from build123d import *

# Parameters (mm, degrees)
SKETCH_W          = 20
SKETCH_H          = 9
PAD_DEPTH         = 0.5
PAD001_DEPTH      = 3
PAD001_FACE6_W    = 9
PAD001_FACE6_H    = 0.5
PAD002_DEPTH      = 160
PAD003_DEPTH      = 3
SKETCH003_R       = 1.7
POCKET_DEPTH      = 5
SKETCH004_W       = 9
SKETCH004_H       = 3.5
POCKET001_DEPTH   = 10
SKETCH005_W       = 9
SKETCH005_H       = 3.5
POCKET002_DEPTH   = 5
POCKET002_FACE2_W = 9
POCKET002_FACE2_H = 165
POCKET002_FACE2_R = 1.7
POCKET003_DEPTH   = 0.1
POCKET004_DEPTH   = 0.1
SKETCH006_R       = 1.9
POCKET005_DEPTH   = 5
POCKET005_FACE6_W = 164.9
POCKET005_FACE6_H = 0.4
POCKET006_DEPTH   = 0.1
POCKET006_FACE1_W = 164.9
POCKET006_FACE1_H = 0.4
POCKET007_DEPTH   = 0.1
POCKET008_DEPTH   = 5


with BuildPart() as part:
    # Sketch → Pad (new body)
    with BuildSketch(Plane.XY):
        Rectangle(SKETCH_W, SKETCH_H)
    extrude(amount=PAD_DEPTH)

    # Sketch001 (on Face6 of Pad) → Pad001 (join)
    with BuildSketch(Plane.XY.offset(0.5)):
        with BuildLine():
            ThreePointArc((-3.6, 2.4), (-6, 0), (-3.6, -2.4))
            Line((-3.6, -2.4), (3.6, -2.4))
            ThreePointArc((3.6, -2.4), (6, 0), (3.6, 2.4))
            Line((-3.6, 2.4), (3.6, 2.4))
        make_face()
    extrude(amount=PAD001_DEPTH)

    # Pad001 Face6 → Pad002 (add)
    with BuildSketch(Plane(origin=(10, 0, 0.25), x_dir=(0, -1, 0), z_dir=(1, 0, 0))):
        Rectangle(PAD001_FACE6_W, PAD001_FACE6_H)
    extrude(amount=PAD002_DEPTH)

    # Sketch002 (on Face6 of Pad002) → Pad003 (join)
    with BuildSketch(Plane.XY.offset(0.5)):
        with BuildLine():
            ThreePointArc((16.6, 2.4), (14.2, 0), (16.6, -2.4))
            Line((16.6, -2.4), (43.8, -2.4))
            ThreePointArc((43.8, -2.4), (46.2, 0), (43.8, 2.4))
            Line((16.6, 2.4), (43.8, 2.4))
        make_face()
        with BuildLine():
            ThreePointArc((56.74, 2.4), (54.34, 0), (56.74, -2.4))
            Line((56.74, -2.4), (83.94, -2.4))
            ThreePointArc((83.94, -2.4), (86.34, 0), (83.94, 2.4))
            Line((56.74, 2.4), (83.94, 2.4))
        make_face()
        with BuildLine():
            ThreePointArc((96.88, 2.4), (94.48, 0), (96.88, -2.4))
            Line((96.88, -2.4), (124.08, -2.4))
            ThreePointArc((124.08, -2.4), (126.48, 0), (124.08, 2.4))
            Line((96.88, 2.4), (124.08, 2.4))
        make_face()
        with BuildLine():
            ThreePointArc((137.02, 2.4), (134.62, 0), (137.02, -2.4))
            Line((137.02, -2.4), (164.22, -2.4))
            ThreePointArc((164.22, -2.4), (166.62, 0), (164.22, 2.4))
            Line((137.02, 2.4), (164.22, 2.4))
        make_face()
    extrude(amount=PAD003_DEPTH)

    # Sketch003 (on Face5 of Pad003) → Pocket (cut)
    with BuildSketch(Plane.XY.offset(0.5)):
        with Locations((10, 0)):
            Circle(SKETCH003_R)
        with Locations((50.1, 0)):
            Circle(SKETCH003_R)
        with Locations((90.2, 0)):
            Circle(SKETCH003_R)
        with Locations((130.3, 0)):
            Circle(SKETCH003_R)
    extrude(amount=-POCKET_DEPTH, mode=Mode.SUBTRACT)

    # Sketch004 (on Face1 of Pocket) → Pocket001 (cut)
    with BuildSketch(Plane(origin=(-10, 0, 0), x_dir=(0, -1, 0), z_dir=(-1, 0, 0))):
        with Locations((0, 1.75)):
            Rectangle(SKETCH004_W, SKETCH004_H)
    extrude(amount=-POCKET001_DEPTH, mode=Mode.SUBTRACT)

    # Sketch005 (on Face3 of Pocket001) → Pocket002 (cut)
    with BuildSketch(Plane.YZ.offset(170)):
        with Locations((0, 1.75)):
            Rectangle(SKETCH005_W, SKETCH005_H)
    extrude(amount=-POCKET002_DEPTH, mode=Mode.SUBTRACT)

    # Pocket002 Face2 → Pocket003 (cut)
    with BuildSketch(Plane(origin=(82.8096, 0, 0), x_dir=(0, -1, 0), z_dir=(0, 0, -1))):
        with Locations((0, 0.3096)):
            Rectangle(POCKET002_FACE2_W, POCKET002_FACE2_H)
        with Locations((0, -47.4904)):
            Circle(POCKET002_FACE2_R, mode=Mode.SUBTRACT)
        with Locations((0, -7.3904)):
            Circle(POCKET002_FACE2_R, mode=Mode.SUBTRACT)
        with Locations((0, 32.7096)):
            Circle(POCKET002_FACE2_R, mode=Mode.SUBTRACT)
        with Locations((0, 72.8096)):
            Circle(POCKET002_FACE2_R, mode=Mode.SUBTRACT)
    extrude(amount=-POCKET003_DEPTH, mode=Mode.SUBTRACT)

    # Pocket003 Face5 → Pocket004 (cut)
    with BuildSketch(Plane(origin=(0, 0, 1.66), x_dir=(0, 1, 0), z_dir=(-1, 0, 0))):
        Polygon((4.5, 1.56), (-4.5, 1.56), (-4.5, 1.16), (-2.4, 1.16), (-2.4, -1.84), (2.4, -1.84), (2.4, 1.16), (4.5, 1.16), align=None)
    extrude(amount=-POCKET004_DEPTH, mode=Mode.SUBTRACT)

    # Sketch006 (on Face12 of Pocket004) → Pocket005 (cut)
    with BuildSketch(Plane.XY.offset(3.5)):
        with Locations((150.3, 0)):
            Circle(SKETCH006_R)
    extrude(amount=-POCKET005_DEPTH, mode=Mode.SUBTRACT)

    # Pocket005 Face6 → Pocket006 (cut)
    with BuildSketch(Plane(origin=(82.55, -4.5, 0.3), x_dir=(-1, 0, 0), z_dir=(0, -1, 0))):
        Rectangle(POCKET005_FACE6_W, POCKET005_FACE6_H)
    extrude(amount=-POCKET006_DEPTH, mode=Mode.SUBTRACT)

    # Pocket006 Face1 → Pocket007 (cut)
    with BuildSketch(Plane(origin=(82.55, 4.5, 0.3), x_dir=(1, 0, 0), z_dir=(0, 1, 0))):
        Rectangle(POCKET006_FACE1_W, POCKET006_FACE1_H)
    extrude(amount=-POCKET007_DEPTH, mode=Mode.SUBTRACT)

    # Sketch007 (on Face16 of Pocket007) → Pocket008 (cut)
    with BuildSketch(Plane.XY.offset(3.5)):
        with BuildLine():
            ThreePointArc((148.8, 1.9), (146.9, 0), (148.8, -1.9))
            Line((148.8, -1.9), (151.8, -1.9))
            ThreePointArc((151.8, -1.9), (153.7, 0), (151.8, 1.9))
            Line((148.8, 1.9), (151.8, 1.9))
        make_face()
    extrude(amount=-POCKET008_DEPTH, mode=Mode.SUBTRACT)


solid = part.part
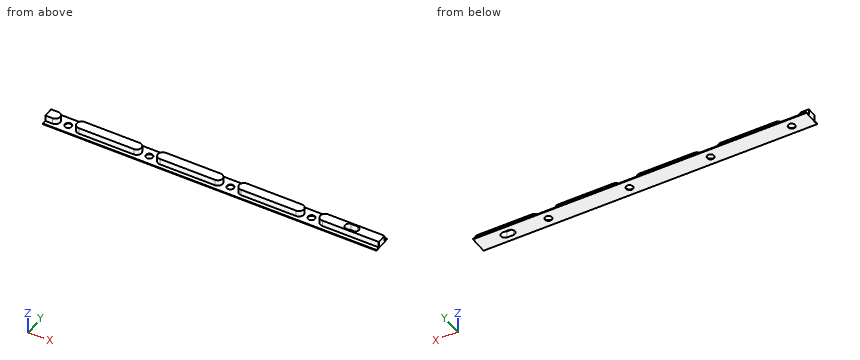
CAD build for the part. Positions are in the model's coordinates, mm. Round coordinates to 2 decimals unless told otherwise and drop trailing zeros. Order: outer loops, then holes, each group sorted by start corner. A loop starts at its lowest first (then second) coordinate and runs counter-clockwise, first axis right, second up. Notation, with made-up numbers: (-8, -13.75) - (19, -13.75) arc R30 cw to (19, 24.25) - close; hole circle Ø8 at (44.5, 54.25). An arc over 180 degrees is marked (long way). Return JSON: item names as keys, results as strings.
(1) Wall check: probe 1 along Y at (x, z) = (10, 0.35); probe 2 along X at (y, z) = (-2, 1.65); probe 3 along Y at (x, z) = (112, 1.6). Give the ranges that are in metal, low to high. Write a range as from..to.
Answer key:
{"probe 1": "y = -4.4..-1.7, 1.7..4.4", "probe 2": "x = 0.1..4.93, 15.27..45.13, 55.41..85.27, 95.55..125.41, 135.69..165", "probe 3": "y = -2.4..2.4"}
(2) Cut at D-D (y = 0). State how many separate pieces and enclosed holes the cut face has, then the cut area to 3 significant figures.
Answer key:
{"separate pieces": "6", "enclosed holes": "0", "area": "434 mm^2"}
(3) Pin check, flat tips, straight feed: pin 1 Ø0.9 at (x, z) = (149.5, 1.5) entering from +Y; pin 2 Ø0.9 at (x, z) = (104, 2.5) entering from -Y. Stop position of each tip, or through.
Answer key:
{"pin 1": "stops at y = 2.4", "pin 2": "stops at y = -2.4"}
(4) Cut at C-C (x = 28.5). Give the cut face in (y, z), then the cut area to 3 significant figures.
Answer key:
{"outline": "(-4.4, 0.1) - (4.4, 0.1) - (4.4, 0.5) - (2.4, 0.5) - (2.4, 3.5) - (-2.4, 3.5) - (-2.4, 0.5) - (-4.4, 0.5) - close", "area": "17.9 mm^2"}
(5) Cut at A-A (z = 2.8). Give the cut face in (x, y).
Answer key:
{"outline": "(0.1, -2.4) - (3.6, -2.4) arc R2.4 ccw to (3.6, 2.4) - (0.1, 2.4) - close; (16.6, -2.4) - (43.8, -2.4) arc R2.4 ccw to (43.8, 2.4) - (16.6, 2.4) arc R2.4 ccw to start; (56.74, -2.4) - (83.94, -2.4) arc R2.4 ccw to (83.94, 2.4) - (56.74, 2.4) arc R2.4 ccw to start; (96.88, -2.4) - (124.08, -2.4) arc R2.4 ccw to (124.08, 2.4) - (96.88, 2.4) arc R2.4 ccw to start; (137.02, -2.4) - (164.22, -2.4) arc R2.4 ccw to (165, -2.27) - (165, 2.27) arc R2.4 ccw to (164.22, 2.4) - (137.02, 2.4) arc R2.4 ccw to start; hole (148.8, -1.9) - (151.8, -1.9) arc R1.9 ccw to (151.8, 1.9) - (148.8, 1.9) arc R1.9 ccw to start"}
(6) Cut at B-B (x = 130.3). Give the cut face in (y, z).
Answer key:
{"outline": "(-4.4, 0.1) - (-1.7, 0.1) - (-1.7, 0.5) - (-4.4, 0.5) - close; (1.7, 0.1) - (4.4, 0.1) - (4.4, 0.5) - (1.7, 0.5) - close"}
